```python
from build123d import *

# Parameters (mm, degrees)
F0_W     = 200
F0_H     = 47.349059
F0_R     = 2.5
F1_DEPTH = 25
F2_R     = 6.804823
F3_DEPTH = 42.8
F4_R     = 4
F5_DEPTH = 42.8


with BuildPart() as f1:
    # F0 (on Top) → F1 (new body)
    with BuildSketch(Plane.XY):
        with Locations((78.801886, -10.301887)):
            Rectangle(F0_W, F0_H)
        with Locations((78.801886, -11.689553)):
            Circle(F0_R, mode=Mode.SUBTRACT)
        with Locations((168.801886, -15.438692)):
            Circle(F0_R, mode=Mode.SUBTRACT)
    extrude(amount=F1_DEPTH)

    # F2 (on face) → F3 (join)
    with BuildSketch(Plane.YZ.offset(178.801886)):
        with Locations((0, 12.338707)):
            Circle(F2_R)
    extrude(amount=F3_DEPTH)

    # F4 (on face) → F5 (cut, through all)
    with BuildSketch(Plane.YZ.offset(221.601886)):
        with Locations((0, 12.338707)):
            Circle(F4_R)
    extrude(amount=-F5_DEPTH, mode=Mode.SUBTRACT)


solid = f1.part
```
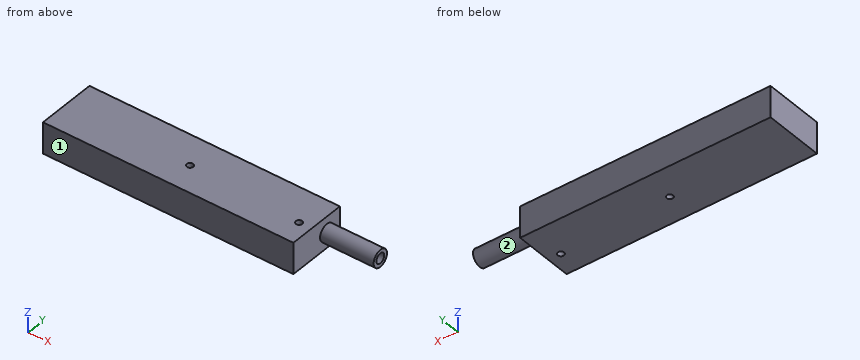
Could you check a few things on this model? Use its own coordinates, in mm. Face numbers are marked on the shaded views. A direction names the side the tool comes from. Round coordinates to 2 decimals unless told otherwise and drop trailing zeros. Loops run counter-clockwise (first coordinate to the right, second up) from the corner with the lowest first, then second, coordinate; pieces in that order, holes last.
Q1. I want a section at A-A (y = 0). Write out the boundary of the cut face in (x, z).
Q2. I want a section at B-B (x = 207). Write out the boundary of the cut face in (y, z), and give its area (3 significant figures).
Q3. Please list where these lines run through material, in increasing order: L1, parallel to Z at x = 213.5, y = 0; L2, parallel to X at y = -21.5, z = 17.5; L3, parallel to X at y = -9.5, z = 17.25.
Q4. I want a section at C-C (y = -20). Write out the boundary of the cut face in (x, z).
Q5. For P1, Ø4.5, axis at x = 168.8, y = -15.44, coming from the +Z side; P2, Ø10, axis at y = -22, z = 20, coming from the +X side; P3, Ø6.5, axis at y = 0.5, z = 11, coming from the +X side, each with a flat end and sliding along its axis, tell me the tip position at first contact or that it passes through.
Q6. On a 3-axis mill with a long thin cutter (end or side, diameter ignored), from which of +Z, -Z, +X, -X, +Y, -Y can I reach the whole of each face in a straight line? I mean the marked faces 1 and 2. Say none if no direction works.
Answer below:
1. outline: (-21.2, 0) - (178.8, 0) - (178.8, 5.53) - (221.6, 5.53) - (221.6, 8.34) - (178.8, 8.34) - (178.8, 16.34) - (221.6, 16.34) - (221.6, 19.14) - (178.8, 19.14) - (178.8, 25) - (-21.2, 25) - close
2. outline: circle Ø13.61 at (0, 12.34); hole circle Ø8 at (0, 12.34)
2. area: 95.2 mm2
3. L1: z = 5.53 to 8.34, 16.34 to 19.14
3. L2: x = -21.2 to 178.8
3. L3: x = -21.2 to 77.6, 80.01 to 178.8
4. outline: (-21.2, 0) - (178.8, 0) - (178.8, 25) - (-21.2, 25) - close
5. P1: passes through
5. P2: stops at x = 178.8
5. P3: stops at x = 221.6
6. face 1: +Z, -Z, +X, -X, -Y
6. face 2: +X
